Part model, mm, in its own coordinate system. A direction names the side the tool comes from. Coordinates: 2 decimals unless noted, no trailing zeros. Loops run counter-clockwise (first coordinate to the right, second up) from the corner with the lowest first, then second, coordinate; pieces in that order, holes last. Notation, with made-up numbers: M 18,-4 L 41,-4 A16 cw 41,27 Z; hole C 16.25,83 d8. An arc over 180 degrees is marked long. Use CSV: the item, a comma, the result in double quotes. Start each with the question number.
from build123d import *

# Parameters (mm, degrees)
F0_R     = 11.5
F1_DEPTH = 5
F2_R     = 10
F3_DEPTH = 11
F4_R     = 11
F5_DEPTH = 2
F6_SIZE  = 1.5
F7_SIZE  = 1.5
F9_DEPTH = 8


with BuildPart() as f1:
    # F0 (on Front) → F1 (new body)
    with BuildSketch(Plane.XZ):
        Circle(F0_R)
    extrude(amount=F1_DEPTH)

    # F2 (on face) → F3 (join)
    with BuildSketch(Plane(origin=(0, 0, 0), x_dir=(-1, 0, 0), z_dir=(0, 1, 0))):
        Circle(F2_R)
    extrude(amount=F3_DEPTH)

    # F4 (on face) → F5 (join)
    with BuildSketch(Plane(origin=(0, 11, 0), x_dir=(-1, 0, 0), z_dir=(0, 1, 0))):
        Circle(F4_R)
    extrude(amount=F5_DEPTH)

    # F6
    f6_edges = [f1.edges().sort_by_distance(p)[0] for p in [
        (11, 13, 0),
    ]]
    chamfer(f6_edges, length=F6_SIZE)

    # F7
    f7_edges = [f1.edges().sort_by_distance(p)[0] for p in [
        (-11.5, -5, 0),
    ]]
    chamfer(f7_edges, length=F7_SIZE)

    # F8 (on face) → F9 (cut)
    with BuildSketch(Plane(origin=(0, 13, 0), x_dir=(-1, 0, 0), z_dir=(0, 1, 0))):
        with BuildLine():
            Line((-8.077747, 5), (-17.5, 5))
            Line((-17.5, 5), (-17.5, -5))
            Line((-17.5, -5), (-8.077747, -5))
            ThreePointArc((-8.077747, -5), (-9.5, 0), (-8.077747, 5))
        make_face()
        with BuildLine():
            Line((17.5, 5), (8.077747, 5))
            ThreePointArc((8.077747, 5), (9.137522, 2.599173), (9.5, 0))
            ThreePointArc((9.5, 0), (9.137522, -2.599173), (8.077747, -5))
            Line((8.077747, -5), (17.5, -5))
            Line((17.5, -5), (17.5, 5))
        make_face()
        with BuildLine():
            Line((-4.898979, 5), (-8.077747, 5))
            ThreePointArc((-8.077747, 5), (-9.5, 0), (-8.077747, -5))
            Line((-8.077747, -5), (-4.898979, -5))
            ThreePointArc((-4.898979, -5), (0, -7), (4.898979, -5))
            Line((4.898979, -5), (8.077747, -5))
            ThreePointArc((8.077747, -5), (9.137522, -2.599173), (9.5, 0))
            ThreePointArc((9.5, 0), (9.137522, 2.599173), (8.077747, 5))
            Line((8.077747, 5), (4.898979, 5))
            ThreePointArc((4.898979, 5), (0, 7), (-4.898979, 5))
        make_face()
    extrude(amount=-F9_DEPTH, mode=Mode.SUBTRACT)


solid = f1.part
1. Wall check: probe 1 along X at (y, z) = (10.75, 5.25); probe 2 along Y at (x, z) = (-5.5, 2.25); probe 3 along Z at (x, y) = (1.75, 10.5). Give the ranges that are in metal, low to high.
2. Slice it at A-A, the plane y = 7.5. List the corners of the cut face in (x, z).
3. Tool access for faces 5 (the face through (-9, 0, 5)), 6 (the face through (0, 11, 10.2)), 7 (the face through (7, 9, 5)), 8 (the face through (0, 11, -10.2)): list every direction of +Z, -Z, +X, -X, +Y, -Y with a clear straight run to the whole face (end or side of a thin tool).
4. Slice it at C-C, the plane z = 0. List the corners of the cut face in (x, y), and give its area (3 significant figures).
5. Slice it at B-B, the plane x = 0. List the corners of the cut face in (y, z), and give its area (4 significant figures).
6. Two-plate mould, pull along Z, no slides. Class faces 1 (the face through (-0.2, 11.2, 11)), 2 (the face through (10, 4, 0)), 3 (the face through (0.2, 11.2, -11)), 4 (the face through (-7, 9, -5)): pulls with the +Z half, pulls with the -Z half, needs draft (parallel to the pull), parting line crosses it, or undercut.
7. Slice it at D-D, the plane y = -1.5. List the corners of the cut face in (x, z).
8. Pin check, flat tips, straight feed: pin 1 (2 mm diameter, centred on y = 0, z = -3.5, fed in from +X) (3 decimals); pin 2 (6 mm diameter, centred on x = 6, y = -1, fed in from +Z); pin 3 (7 mm diameter, centred on x = 5.5, z = -0.5, fed in from +Y). Stop position of each tip, or through.
Found:
1,probe 1,"-8.51 to -4.63, 4.63 to 8.51"
1,probe 2,"-5 to 5"
1,probe 3,"-9.85 to -6.78, 6.78 to 9.85"
2,outline,"M -8.66,-5 A10 ccw 8.66,-5 L 4.9,-5 A7 cw -4.9,-5 Z; M -8.66,5 L -4.9,5 A7 cw 4.9,5 L 8.66,5 A10 ccw Z"
3,face 5,"none"
3,face 6,"+Z"
3,face 7,"+X, -X, +Y"
3,face 8,"-Z"
4,outline,"M -11.5,-3.5 L -10,-5 L 10,-5 L 11.5,-3.5 L 11.5,0 L 10,0 L 10,5 L -10,5 L -10,0 L -11.5,0 Z"
4,area,"213 mm^2"
5,outline,"M -5,-10 L -3.5,-11.5 L 0,-11.5 L 0,-10 L 11,-10 L 11,-11 L 11.5,-11 L 13,-9.5 L 13,-7 L 5,-7 L 5,7 L 13,7 L 13,9.5 L 11.5,11 L 11,11 L 11,10 L 0,10 L 0,11.5 L -3.5,11.5 L -5,10 Z"
5,area,"262.5 mm^2"
6,face 1,"pulls with the +Z half"
6,face 2,"parting line crosses it"
6,face 3,"pulls with the -Z half"
6,face 4,"undercut"
7,outline,"C 0,0 d23"
8,pin 1,"x = 11.225"
8,pin 2,"z = 11.1"
8,pin 3,"y = 5"
